Geometry check sheet. Reference: drawing and pictorial views, mm from the part's lowest x, y, z. A direction names the side the tool comes from. Round coordinates to 2 decimals unless told otherwise and drop trailing zeros.
(1) Material ranges on line 1 along X through (y, z) = (2.85, 6.35); line 2 along Y through (x, z) = (9.5, 1); line 3 along X through (y, z) = (2.5, 7), recorded low to high.
(2) Go/stop test with flat-tipped pins: pin 1 (5 mm diameter, centred on x = 6, z = 4.5, fed in from +Y); pin 2 (1.5 mm diameter, centred on y = 5.5, z = 5.5, fed in from +X); pin 3 (5.5 mm diameter, centred on x = 6.35, z = 6.35, fed in from -Y); pin 4 (4 mm diameter, centred on y = 5.5, z = 6, fed in from +X). Record where each tip stops, or that it passes through.
(3) Set-up check for the marked faces 4 and 5: record each of +Z, -Z, +X, -X, +Y, -Y from which the full face is reachable in a straight line by a thin tool's end or side.
(4) Release check for a two-part mould opening along X. For the marked faces 1, 2 and 3 record: +X half, -X half, draft (parallel to the pull), parting line (faces both ways), or undercut.
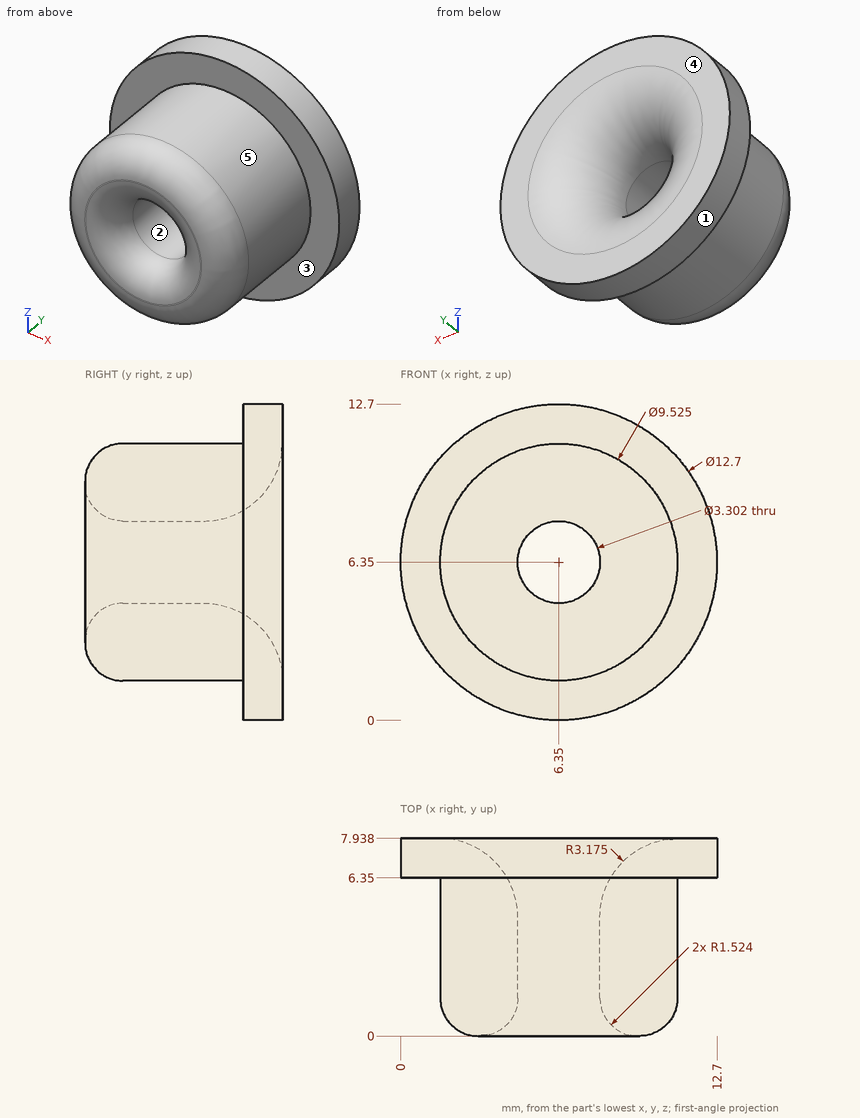
Answer below:
1. line 1: x = 1.59 to 4.7, 8 to 11.11
1. line 2: y = 6.35 to 7.94
1. line 3: x = 1.63 to 4.83, 7.87 to 11.07
2. pin 1: stops at y = 7.91
2. pin 2: stops at x = 11.11
2. pin 3: stops at y = 0.06
2. pin 4: stops at x = 12.7
3. face 4: +Z, -Z, +X, -X, +Y
3. face 5: -Y
4. face 1: parting line
4. face 2: undercut
4. face 3: draft
